```python
from build123d import *

# Parameters (mm, degrees)
SKIZZE1_W                       = 52.482326825
SKIZZE1_H                       = 22.353583648
AUFSATZ_LINEAR_AUSTRAGEN1_DEPTH = 200
FASE1_SIZE                      = 10


with BuildPart() as part:
    # Skizze1 → Aufsatz-Linear austragen1 (new body)
    with BuildSketch(Plane.XY):
        with Locations((-162.31044063, 135.449774465)):
            Rectangle(SKIZZE1_W, SKIZZE1_H)
    extrude(amount=AUFSATZ_LINEAR_AUSTRAGEN1_DEPTH)

    # Fase1
    fase1_edges = [part.edges().sort_by_distance(p)[0] for p in [
        (-136.069277217, 146.626566289, 100),
    ]]
    chamfer(fase1_edges, length=FASE1_SIZE)


solid = part.part
```
Can you work these out from the model? Positions are in its coordinate system, mm. Coordinates: 2 decimals unless noted, no trailing zeros. Loops run counter-clockwise (first coordinate to the right, second up) from the corner with the lowest first, then second, coordinate; pieces in that order, holes last. Notation, with made-up numbers: (78.25, 64.5) - (128.25, 64.5) arc R16 cw to (128.25, 76.5) - close; hole circle Ø4 at (23.5, 43). An arc over 180 degrees is marked (long way). Use a Markdown table: item, result.
Item 1: Will this pin go through, and if not, where does the flat tip stop? pin 1 (12 mm diameter, centred on x = -146, y = 140, fed in from -Z).
Numbers:
| item | result |
|---|---|
| pin 1 | stops at z = 0 |
Item 2: I want a section at B-B on y = 142.25. Please give me the cut outline in (x, z).
Numbers:
| item | result |
|---|---|
| outline | (-188.55, 0) - (-141.69, 0) - (-141.69, 200) - (-188.55, 200) - close |
Item 3: I want a section at C-C on x = -141. Please give me the cut outline in (y, z).
Numbers:
| item | result |
|---|---|
| outline | (124.27, 0) - (141.56, 0) - (141.56, 200) - (124.27, 200) - close |
Item 4: If I drill on probe 1 along X at (y, z) = (142, 158); probe 2 along X at (y, z) = (140, 65.5); probe 3 along Y at (x, z) = (-141, 53.5), over which ranges is the centre line in solid material (lowest first)? Write a range as from..to.
Numbers:
| item | result |
|---|---|
| probe 1 | x = -188.55..-141.44 |
| probe 2 | x = -188.55..-139.44 |
| probe 3 | y = 124.27..141.56 |
Item 5: I want a section at A-A on z = 93. Please give me the cut outline in (x, y).
Numbers:
| item | result |
|---|---|
| outline | (-188.55, 124.27) - (-136.07, 124.27) - (-136.07, 136.63) - (-146.07, 146.63) - (-188.55, 146.63) - close |
